Model file for the job. Use its own axes, mm. A direction names the side the tool comes from. Give positions to 0.01 mm unless a question says otherwise; leave off trailing zeros. Write each loop counter-clockwise with the first axis right and the second up, starting at its lowest first coordinate (ties: lowest second). Pieces come first, ordered by that corner, then holes. Notation, with made-up numbers: (61.5, 16.25) - (87.5, 16.25) arc R20 ccw to (87.5, 26.25) - close; hole circle Ø10 at (65, -14.5). An arc over 180 degrees is marked (long way). One line per item, written item: value. Start each with the question number.
(1) Cut at A-A, the plane z = 3.5. List the corners of the cut face in (x, y), and give its area (3 significant figures).
(2) Cut at B-B, the plane x = -5.5. List the corners of the cut face in (y, z), and give its area (3 significant figures).
(3) Drop a flat-ended pin along its axis: P1, Ø2, axis at x = -5.5, y = 1.5, coming from the +Z side. Give the stop position or say it passes through.
(4) Cut at C-C, the plane y = -9. List the corners of the cut face in (x, z), and give its area (3 significant figures).
(5) Probe L1, parallel to Y at x = 3, z = 13.5; L2, parallel to Z at x = -4.25, y = -5. List the from-to ranges inside material, lowest first.
(6) 3-axis set-ups, long thin cutter, end or side, ignore diameter. For faces 1 (the face through (7.5, 0.9, -0.7)), 2 (the face through (0, 10.25, 8)): which of +Z, -Z, +X, -X, +Y, -Y reach the whole face in a straight line?
(7) Mould opens along Y. For faces 3 (the face through (0.11, 10.73, -0.5)), 4 (the face through (0, -11.25, 8)), 5 (the face through (0, -10.25, 8)) say: pulls with the +Y half, pulls with the -Y half, needs draft (parallel to the pull), parting line crosses it, or undercut.
from build123d import *

# Parameters (mm, degrees)
SKETCH1_W                    = 15
SKETCH1_H                    = 20
BASE_FLANGE1_DEPTH           = 1
EDGE_FLANGE1_STRIP_W         = 5.7232
EDGE_FLANGE1_STRIP_H         = 1
EDGE_FLANGE1_STRIP_CUT_DEPTH = 15
EDGE_FLANGE1_DEPTH           = 15
EDGE_FLANGE2_STRIP_W         = 5.7232
EDGE_FLANGE2_STRIP_H         = 1
EDGE_FLANGE2_STRIP_CUT_DEPTH = 15
EDGE_FLANGE2_DEPTH           = 15


# Sheet-metal steps are written as plain solids
with BuildPart() as part:
    # Sketch1 → Base-Flange1 (new body)
    with BuildSketch(Plane.XY):
        Rectangle(SKETCH1_W, SKETCH1_H)
    extrude(amount=-BASE_FLANGE1_DEPTH)

    # Edge-Flange1 strip (across the edge) → Edge-Flange1 strip cut (cut)
    with BuildSketch(Plane(origin=(7.5, 10.25, 0), x_dir=(0, -1, 0), z_dir=(-1, 0, 0))):
        with Locations((-2.125, -0.5)):
            Rectangle(EDGE_FLANGE1_STRIP_W, EDGE_FLANGE1_STRIP_H)
    extrude(amount=EDGE_FLANGE1_STRIP_CUT_DEPTH, mode=Mode.SUBTRACT)

    # Edge-Flange1 section (across the edge) → Edge-Flange1 (add)
    with BuildSketch(Plane(origin=(7.5, 10.25, 0), x_dir=(0, -1, 0), z_dir=(-1, 0, 0))):
        with BuildLine():
            Line((-1, 0.7366), (-1, 15))
            Line((-1, 15), (0, 15))
            Line((0, 15), (0, 0.7366))
            ThreePointArc((0, 0.7366), (0.215745145, 0.215745145), (0.7366, 0))
            Line((0.7366, 0), (0.7366, -1))
            ThreePointArc((0.7366, -1), (-0.491361636, -0.491361636), (-1, 0.7366))
        make_face()
    extrude(amount=EDGE_FLANGE1_DEPTH)

    # Edge-Flange2 strip (across the edge) → Edge-Flange2 strip cut (cut)
    with BuildSketch(Plane(origin=(-7.5, -10.25, 0), x_dir=(0, 1, 0), z_dir=(1, 0, 0))):
        with Locations((-2.125, -0.5)):
            Rectangle(EDGE_FLANGE2_STRIP_W, EDGE_FLANGE2_STRIP_H)
    extrude(amount=EDGE_FLANGE2_STRIP_CUT_DEPTH, mode=Mode.SUBTRACT)

    # Edge-Flange2 section (across the edge) → Edge-Flange2 (add)
    with BuildSketch(Plane(origin=(-7.5, -10.25, 0), x_dir=(0, 1, 0), z_dir=(1, 0, 0))):
        with BuildLine():
            Line((-1, 0.7366), (-1, 15))
            Line((-1, 15), (0, 15))
            Line((0, 15), (0, 0.7366))
            ThreePointArc((0, 0.7366), (0.215745145, 0.215745145), (0.7366, 0))
            Line((0.7366, 0), (0.7366, -1))
            ThreePointArc((0.7366, -1), (-0.491361636, -0.491361636), (-1, 0.7366))
        make_face()
    extrude(amount=EDGE_FLANGE2_DEPTH)


solid = part.part
Answers follow:
1. outline: (-7.5, -11.25) - (7.5, -11.25) - (7.5, -10.25) - (-7.5, -10.25) - close; (-7.5, 10.25) - (7.5, 10.25) - (7.5, 11.25) - (-7.5, 11.25) - close
1. area: 30.0 mm²
2. outline: (-11.25, 0.74) arc R1.74 ccw to (-9.51, -1) - (9.51, -1) arc R1.74 ccw to (11.25, 0.74) - (11.25, 15) - (10.25, 15) - (10.25, 0.74) arc R0.74 cw to (9.51, 0) - (-9.51, 0) arc R0.74 cw to (-10.25, 0.74) - (-10.25, 15) - (-11.25, 15) - close
2. area: 51.4 mm²
3. P1: stops at z = 0
4. outline: (-7.5, -1) - (7.5, -1) - (7.5, 0) - (-7.5, 0) - close
4. area: 15.0 mm²
5. L1: y = -11.25 to -10.25, 10.25 to 11.25
5. L2: z = -1 to 0
6. face 1: +Z, -Z, +X, +Y, -Y
6. face 2: +Z, +X, -X
7. face 3: pulls with the +Y half
7. face 4: pulls with the -Y half
7. face 5: undercut
